Design review of the part built by this model. Coordinates are the model's own, in mm. A direction names the side the tool comes from. Round coordinates to 2 decimals unless told otherwise and drop trailing zeros. Order: outer loops, then holes, each group sorted by start corner. A loop starts at its lowest first (then second) coordinate and runs counter-clockwise, first axis right, second up. Notation, with made-up numbers: M 42,-35.5 L 93,-35.5 A19 ccw 93,-29.5 Z; hole C 71.5,12 d1. An arc over 180 degrees is marked long. Write each question's results on one line, items separated by ' | '. Start each with the question number.
Item 1: Machinability: for faces 1 (the cylindrical face through (-7.215, -2.36, 4.699)), 2 (the cylindrical face through (7.215, -2.64, 4.699)), 3 (the flat face through (0, -10, 25)), which of the approach directions +Z, -Z, +X, -X, +Y, -Y give a long, thin tool a straight path to every point of the face, cutting with its end or side? Answer none if there is none.
Item 2: Clearance check with flat-ended pins moving along their axes: pin 1 (2.5 mm diameter, centred on x = 0, y = 7.5, fed in from -Z); pin 2 (6.5 mm diameter, centred on x = -2.5, y = 5, fed in from +Z); pin 3 (1 mm diameter, centred on x = -5.5, y = -16, fed in from -Z); pin 4 (3 mm diameter, centred on x = -0.5, z = 16, fed in from +Y). State where each tip first meets the part, or that it passes through.
Item 3: The part is to be moulded in two halves that separate along Z. For faces 4 (the flat face through (0, 0, 0)), 5 (the cylindrical face through (-7.215, -10.035, 25.301)), 6 (the cylindrical face through (0.035, 12.215, 4.699)), 7 (the cylindrical face through (6, 11.07, 2.48)), say which applies: +Z half, -Z half, draft (parallel to the pull), parting line (faces both ways), or undercut.
Item 4: Wall thickness on line 1 (Z direction, x = 4.25, y = -11); line 2 (X direction, y = 7.5, z = 2.5); line 3 (Z direction, x = -4.75, y = 6): over which ranges is each line inside the solid? List them lowest first. Write a range as [from, to].
Item 5: Take a section at B-B, the plane y = 0.5. Write out the cut boundary in (x, z), plus the area to 3 significant figures.
Item 6: Take a section at A-A, the plane x = 0. Write out the cut boundary in (y, z), plus the area to 3 significant figures.
Item 7: Take a section at C-C, the plane z = 15. Write out the cut boundary in (x, y), plus the area to 3 significant figures.
Autodesk Inventor part; units mm, degrees
ref_plane "YZ Plane" through (0, 0, 0) normal (1, 0, 0) x (0, 1, 0)
ref_plane "XZ Plane" through (0, 0, 0) normal (0, 1, 0) x (-1, 0, 0)
ref_plane "XY Plane" through (0, 0, 0) normal (0, 0, 1) x (1, 0, 0)
sketch "Sketch1" plane through (0, 0, 0) normal (0, 0, 1) x (1, 0, 0)
  line L0 (-2.5, 12.5) -> (2.5, 12.5)
  line L1 (7.5, 7.5) -> (7.5, -12.5)
  line L2 (7.5, -12.5) -> (-7.5, -12.5)
  line L3 (-7.5, -12.5) -> (-7.5, 7.5)
  line L4 (-7.5, 12.5) -> (7.5, -12.5) construction
  line L5 (7.5, 12.5) -> (-7.5, -12.5) construction
  arc A0 (-2.5, 12.5) -> (-7.5, 7.5) centre (-2.5, 7.5) ccw
  arc A1 (7.5, 7.5) -> (2.5, 12.5) centre (2.5, 7.5) ccw
  circle A2 centre (0, 7.5) radius 1.5
  point P0 (0, 0)
  dimension "d0" = 15
  dimension "d3" = 5
  dimension "d4" = 3
  dimension "d5" = 5
  dimension "HOOK_HEIGHT" = 20
extrude "Extrusion2" add sketch "Sketch1" along normal blind 5
sketch "Sketch2" plane through (0, 0, 5) normal (0, 0, 1) x (1, 0, 0)
  circle A0 centre (0, 7.5) radius 1.5
  point P0 (0, 0)
hole "Hole1" at (0, 7.5, 5) direction (0, 0, -1) diameter 4 end through all countersink diameter 6 countersink angle 90
sketch "Sketch3" plane through (-7.5, -12.5, 0) normal (-1, 0, 0) x (0, 0, 1)
  line L0 (0, 0) -> (5, 0)
  line L1 (2.5, 0) -> (2.5, -6.8079) construction
  arc A0 (0, 0) -> (30, 0) centre (15, 0) ccw
  line L2 (5, 20) -> (5, 0) construction
  line L3 (0, 20) -> (0, 0) construction
  arc A1 (5, 0) -> (25, 0) centre (15, 0) ccw
  line L4 (25, 0) -> (25, 5)
  line L5 (30, 5) -> (30, 0)
  arc A2 (30, 5) -> (25, 5) centre (27.5, 5) ccw
  point P0 (0, 12.5)
  dimension "HOOK_RADIUS" = 30
  dimension "d16" = 5
  dimension "HOOK_LEN" = 5
  dimension "d18" = 5
extrude "Extrusion3" add sketch "Sketch3" against normal up to surface (15 mm away)
fillet "Fillet1" radius 1 18 edges at (7.5, -2.5, 5) (6.0355, 11.0355, 5) (0, 12.5, 5) (-6.0355, 11.0355, 5) (-7.5, -2.5, 5) (-7.5, -22.5, 15) (-7.5, -10, 25) (-7.5, -5, 27.5) (-7.5, -10, 30) (-7.5, -27.5, 15) (-7.5, -2.5, 0) (-6.0355, 11.0355, 0) (0, 12.5, 0) (6.0355, 11.0355, 0) (7.5, -2.5, 0) (7.5, -10, 30) (7.5, -5, 27.5) (7.5, -10, 25)
properties part number "curved_single_hook" material "PET Plastic"
Results list:
1) face 1: -X, +Y | face 2: +X, +Y | face 3: +X, -X, +Y
2) pin 1: through | pin 2: z = 5 | pin 3: z = 0.3 | pin 4: y = -22.18
3) face 4: -Z half | face 5: undercut | face 6: +Z half | face 7: draft
4) line 1: [0, 5], [25, 30] | line 2: [-7.5, -2], [2, 7.5] | line 3: [0, 5]
5) outline: M -7.5,1 A1 ccw -6.5,0 L 6.5,0 A1 ccw 7.5,1 L 7.5,4 A1 ccw 6.5,5 L -6.5,5 A1 ccw -7.5,4 Z | area: 74.1 mm²
6) outline: M -12.5,0 L 5.5,0 L 5.5,4 L 4.5,5 L -12.5,5 A10 cw -12.5,25 L -7.5,25 A2.5 ccw -7.5,30 L -12.5,30 A15 ccw Z; M 9.5,0 L 11.5,0 A1 ccw 12.5,1 L 12.5,4 A1 ccw 11.5,5 L 10.5,5 L 9.5,4 Z | area: 335 mm²
7) outline: M -7.5,-26.5 A1 ccw -6.5,-27.5 L 6.5,-27.5 A1 ccw 7.5,-26.5 L 7.5,-23.5 A1 ccw 6.5,-22.5 L -6.5,-22.5 A1 ccw -7.5,-23.5 Z | area: 74.1 mm²
